The model under review builds one solid part; all positions refer to its coordinate system, in mm. Face numbers are marked on the shaded views. A direction names the side the tool comes from. Give positions to 0.01 mm unless a question says otherwise; leave off trailing zeros. Loops run counter-clockwise (first coordinate to the right, second up) from the corner with the lowest first, then second, coordinate; pieces in that order, holes last. Notation, with made-up numbers: M -13,20 L 31,20 A22 cw 31,49 Z; hole C 64.25,14 d2. An arc over 180 degrees is marked long. Return JSON: item names as keys, results as strings.
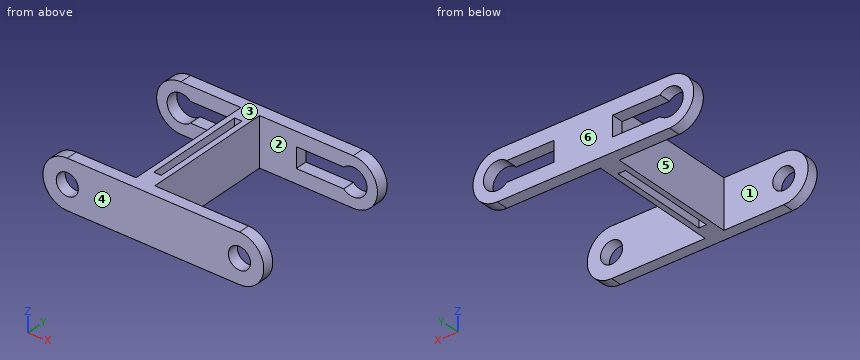
```python
from build123d import *

# Parameters (mm, degrees)
BOSS_EXTRUDE1_START   = 43.1
SKETCH1_R             = 6.5
BOSS_EXTRUDE1_DEPTH   = 1.6
BOSS_EXTRUDE1_2_DEPTH = 1.6
BOSS_EXTRUDE2_START   = 43.1
SKETCH2_W             = 46
SKETCH2_H             = 13
BOSS_EXTRUDE2_DEPTH   = 1.6
CUT_EXTRUDE1_START    = 43.1
SKETCH3_R             = 3.7
CUT_EXTRUDE1_DEPTH    = 1.6
CUT_EXTRUDE2_START    = 43.1
SKETCH4_W             = 15.2
SKETCH4_H             = 5.4
CUT_EXTRUDE2_DEPTH    = 1.6
BOSS_EXTRUDE3_START   = 5
SKETCH5_R             = 6.5
BOSS_EXTRUDE3_DEPTH   = 1.5
BOSS_EXTRUDE3_2_DEPTH = 1.5
BOSS_EXTRUDE4_START   = 5
SKETCH6_W             = 46
SKETCH6_H             = 13
BOSS_EXTRUDE4_DEPTH   = 1.5
CUT_EXTRUDE3_START    = 5
SKETCH7_R             = 2.95
CUT_EXTRUDE3_DEPTH    = 1.5
BOSS_EXTRUDE5_START   = 18.5
SKETCH8_W             = 13
SKETCH8_H             = 41.2
BOSS_EXTRUDE5_DEPTH   = 2.5
CUT_EXTRUDE4_START    = -0.01
SKETCH9_W             = 2
SKETCH9_H             = 27
CUT_EXTRUDE4_DEPTH    = 6.51


with BuildPart() as part:
    # Sketch1 → Boss-Extrude1 (new, symmetric)
    with BuildSketch(Plane(origin=(0, 0, 0), x_dir=(1, 0, 0), z_dir=(0, 1, 0)).offset(BOSS_EXTRUDE1_START)):
        with Locations(Location((0, 0, 0), (0, 0, 270))):
            Circle(SKETCH1_R)
    extrude(amount=BOSS_EXTRUDE1_DEPTH, both=True)



with BuildPart() as body_2:
    # Sketch1 → Boss-Extrude1 2 (new, symmetric)
    with BuildSketch(Plane(origin=(0, 0, 0), x_dir=(1, 0, 0), z_dir=(0, 1, 0)).offset(BOSS_EXTRUDE1_START)):
        with Locations(Location((46, 0, 0), (0, 0, 270))):
            Circle(SKETCH1_R)
    extrude(amount=BOSS_EXTRUDE1_2_DEPTH, both=True)


with BuildPart() as part_1:
    add(part.part)

    add(body_2.part)  # Boss-Extrude2 merges body 2
    # Sketch2 → Boss-Extrude2 (add, symmetric)
    with BuildSketch(Plane(origin=(0, 0, 0), x_dir=(1, 0, 0), z_dir=(0, 1, 0)).offset(BOSS_EXTRUDE2_START)):
        with Locations((23, 0)):
            Rectangle(SKETCH2_W, SKETCH2_H)
    extrude(amount=BOSS_EXTRUDE2_DEPTH, both=True)

    # Sketch3 → Cut-Extrude1 (cut, symmetric)
    with BuildSketch(Plane(origin=(0, 0, 0), x_dir=(1, 0, 0), z_dir=(0, 1, 0)).offset(CUT_EXTRUDE1_START)):
        with Locations(Location((0, 0, 0), (0, 0, 270))):
            Circle(SKETCH3_R)
        with Locations(Location((46, 0, 0), (0, 0, 270))):
            Circle(SKETCH3_R)
    extrude(amount=CUT_EXTRUDE1_DEPTH, both=True, mode=Mode.SUBTRACT)

    # Sketch4 → Cut-Extrude2 (cut, symmetric)
    with BuildSketch(Plane(origin=(0, 0, 0), x_dir=(1, 0, 0), z_dir=(0, 1, 0)).offset(CUT_EXTRUDE2_START)):
        with Locations((7.6, 0)):
            Rectangle(SKETCH4_W, SKETCH4_H)
        with Locations((38.4, 0)):
            Rectangle(SKETCH4_W, SKETCH4_H)
    extrude(amount=CUT_EXTRUDE2_DEPTH, both=True, mode=Mode.SUBTRACT)



with BuildPart() as body_2_2:
    # Sketch5 → Boss-Extrude3 (new, symmetric)
    with BuildSketch(Plane(origin=(0, 0, 0), x_dir=(1, 0, 0), z_dir=(0, 1, 0)).offset(BOSS_EXTRUDE3_START)):
        with Locations(Location((0, 0, 0), (0, 0, 270))):
            Circle(SKETCH5_R)
    extrude(amount=BOSS_EXTRUDE3_DEPTH, both=True)



with BuildPart() as body_3:
    # Sketch5 → Boss-Extrude3 2 (new, symmetric)
    with BuildSketch(Plane(origin=(0, 0, 0), x_dir=(1, 0, 0), z_dir=(0, 1, 0)).offset(BOSS_EXTRUDE3_START)):
        with Locations(Location((46, 0, 0), (0, 0, 270))):
            Circle(SKETCH5_R)
    extrude(amount=BOSS_EXTRUDE3_2_DEPTH, both=True)


with BuildPart() as body_2_2_1:
    add(body_2_2.part)

    add(body_3.part)  # Boss-Extrude4 merges body 3
    # Sketch6 → Boss-Extrude4 (add, symmetric)
    with BuildSketch(Plane(origin=(0, 0, 0), x_dir=(1, 0, 0), z_dir=(0, 1, 0)).offset(BOSS_EXTRUDE4_START)):
        with Locations((23, 0)):
            Rectangle(SKETCH6_W, SKETCH6_H)
    extrude(amount=BOSS_EXTRUDE4_DEPTH, both=True)

    # Sketch7 → Cut-Extrude3 (cut, symmetric)
    with BuildSketch(Plane(origin=(0, 0, 0), x_dir=(1, 0, 0), z_dir=(0, 1, 0)).offset(CUT_EXTRUDE3_START)):
        with Locations(Location((0, 0, 0), (0, 0, 270))):
            Circle(SKETCH7_R)
        with Locations(Location((46, 0, 0), (0, 0, 270))):
            Circle(SKETCH7_R)
    extrude(amount=CUT_EXTRUDE3_DEPTH, both=True, mode=Mode.SUBTRACT)


with BuildPart() as part_2:
    add(part_1.part)

    add(body_2_2_1.part)  # Boss-Extrude5 merges body 2 2
    # Sketch8 → Boss-Extrude5 (add, symmetric)
    with BuildSketch(Plane(origin=(0, 0, 0), x_dir=(0, 0, -1), z_dir=(1, 0, 0)).offset(BOSS_EXTRUDE5_START)):
        with Locations((0, 24.1)):
            Rectangle(SKETCH8_W, SKETCH8_H)
    extrude(amount=BOSS_EXTRUDE5_DEPTH, both=True)

    # Sketch9 → Cut-Extrude4 (cut, symmetric)
    with BuildSketch(Plane.XY.offset(CUT_EXTRUDE4_START)):
        with Locations((18.5, 24)):
            Rectangle(SKETCH9_W, SKETCH9_H)
    extrude(amount=CUT_EXTRUDE4_DEPTH, both=True, mode=Mode.SUBTRACT)


solid = part_2.part
```
1) Consider section B-B on y = 34. Write out the cut boundary in (x, z).
From the geometry:
{"outline": "M 16,-6.5 L 17.5,-6.5 L 17.5,6.5 L 16,6.5 Z; M 19.5,-6.5 L 21,-6.5 L 21,6.5 L 19.5,6.5 Z"}
2) Wall thickness on L1, parallel to X at y = 4.6, z = 0; L2, parallel to X at y = 43.5, z = 0; L3, parallel to X at y = 31.5, z = -1: over which ranges is each line inside the solid? List them lowest first. Write a range as from..to.
From the geometry:
{"L1": "-6.5..-2.95, 2.95..43.05, 48.95..52.5", "L2": "-6.5..-3.7, 15.2..30.8, 49.7..52.5", "L3": "16..17.5, 19.5..21"}
3) Consider section C-C on x = 35.5. Write out the cut boundary in (y, z).
From the geometry:
{"outline": "M 3.5,-6.5 L 6.5,-6.5 L 6.5,6.5 L 3.5,6.5 Z; M 41.5,-6.5 L 44.7,-6.5 L 44.7,-2.7 L 41.5,-2.7 Z; M 41.5,2.7 L 44.7,2.7 L 44.7,6.5 L 41.5,6.5 Z"}
4) Consider section D-D on z = -4.5. Write out the cut boundary in (x, y), then the cut area to 3 significant figures.
From the geometry:
{"outline": "M -4.69,3.5 L 50.69,3.5 L 50.69,6.5 L 21,6.5 L 21,41.5 L 50.69,41.5 L 50.69,44.7 L -4.69,44.7 L -4.69,41.5 L 16,41.5 L 16,6.5 L -4.69,6.5 Z; hole M 17.5,10.5 L 19.5,10.5 L 19.5,37.5 L 17.5,37.5 Z", "area": "464 mm²"}
5) Tool access review of the marked faces 1, 2 and 3: name each direction out of +Z, -Z, +X, -X, +Y, -Y from which nothing blocks a thin tool from reaching the whole face with its end or side.
From the geometry:
{"face 1": "+Z, -Z, -X", "face 2": "+Z, -Z, +X", "face 3": "+Z, +X, -X, +Y, -Y"}
6) Insertion check: pin 1 (5 mm diameter, centred on y = 38, z = 0.5, fed in from -X); pin 2 (4 mm diameter, centred on y = 20, z = 2.5, fed in from +X); pin 3 (4 mm diameter, centred on x = 0, z = 1, fed in from +Y). Each pin has a flat end and moves straight along its axis. Give the tip position at first contact, or say it passes through.
From the geometry:
{"pin 1": "x = 16", "pin 2": "x = 21", "pin 3": "y = 6.5"}
7) The part is to be moulded in two halves that separate along Y. For the marked faces 4, 5 and 6, say which applies: released by +Y, released by -Y, zero draft, split by the parting line, or undercut.
From the geometry:
{"face 4": "released by -Y", "face 5": "undercut", "face 6": "released by +Y"}
8) Consider section A-A on z = 0. Count the separate pieces of the cut face and the enclosed holes in it, then the cut area to 3 significant figures.
From the geometry:
{"separate pieces": "5", "enclosed holes": "1", "area": "330 mm²"}
